from build123d import *

# Parameters (mm, degrees)
BOSS_EXTRUDE1_DEPTH       = 3.175
SKETCH2_R                 = 3.14
BOSS_EXTRUDE2_DEPTH       = 15.04125
F_4_CLEARANCE_HOLE1_D     = 3.2639
F_4_CLEARANCE_HOLE1_DEPTH = 25.4
F_4_CLEARANCE_HOLE1_TIP   = 0.980574487


with BuildPart() as part:
    # Sketch1 → Boss-Extrude1 (new body)
    with BuildSketch(Plane(origin=(0, 0, 0), x_dir=(1, 0, 0), z_dir=(0, 1, 0))):
        Polygon((0, 36.805), (-0.035, 36.805), (-52.035, 36.805), (-52.035, -36.805), (-0.035, -36.805), (0, -36.805), align=None)
    extrude(amount=-BOSS_EXTRUDE1_DEPTH)

    # Sketch2 → Boss-Extrude2 (add)
    with BuildSketch(Plane(origin=(0, 0, 0), x_dir=(1, 0, 0), z_dir=(0, 1, 0))):
        with BuildLine():
            Line((-3.175, 30.2), (0, 30.2))
            Line((0, 30.2), (0, 36.48))
            Line((0, 36.48), (-3.175, 36.48))
            ThreePointArc((-3.175, 36.48), (-6.315, 33.34), (-3.175, 30.2))
        make_face()
        with BuildLine():
            Line((-3.175, -36.48), (0, -36.48))
            Line((0, -36.48), (0, -30.2))
            Line((0, -30.2), (-3.175, -30.2))
            ThreePointArc((-3.175, -30.2), (-6.315, -33.34), (-3.175, -36.48))
        make_face()
        with Locations(Location((-48.895, 33.34, 0), (0, 0, 270))):
            Circle(SKETCH2_R)
        with Locations(Location((-48.895, -33.34, 0), (0, 0, 270))):
            Circle(SKETCH2_R)
    extrude(amount=-BOSS_EXTRUDE2_DEPTH)

    # #4 Clearance Hole1
    with Locations(Plane(origin=(0, -15.04125, 0), x_dir=(-1, 0, 0), z_dir=(0, -1, 0))):
        with Locations((48.895, 33.34), (3.175, 33.34), (3.175, -33.34), (48.895, -33.34)):
            Hole(F_4_CLEARANCE_HOLE1_D / 2, depth=F_4_CLEARANCE_HOLE1_DEPTH)
            with Locations((0, 0, -(F_4_CLEARANCE_HOLE1_DEPTH + F_4_CLEARANCE_HOLE1_TIP / 2))):  # 118° drill point
                Cone(0, F_4_CLEARANCE_HOLE1_D / 2, F_4_CLEARANCE_HOLE1_TIP, mode=Mode.SUBTRACT)

    # Mirror1: part across plane


with BuildPart() as part_1:
    add(part.part)
    add(part.part.mirror(Plane(origin=(0, -3.175, 0), x_dir=(0, 0, 1), z_dir=(-1, 0, 0))))


solid = part_1.part
The model under review builds one solid part; all positions refer to its coordinate system, in mm. A direction names the side the tool comes from. Round coordinates to 2 decimals unless told otherwise and drop trailing zeros. Write each loop counter-clockwise with the first axis right and the second up, starting at its lowest first coordinate (ties: lowest second). Pieces come first, ordered by that corner, then holes. Notation, with made-up numbers: M 83,7 L 136,7 A21 cw 136,39 Z; hole C 68,73 d1. An arc over 180 degrees is marked long. Use a Markdown table: item, result. Add a question column.
Q1. We need section C-C, the plane x = 11.5. State the section outline as (y, z) points (3 decimals).
Q2. The part is to be moulded in two halves that separate along X. For faces 6 (the face through (50.1, -7.42, 32.24)), 7 (the face through (52.035, -2, -1)), 8 (the face through (50.1, -9.03, 36.24)), 9 (the face through (0, -9, -36.48)), say which applies: pulls with the +X half, pulls with the -X half, needs draft (parallel to the pull), parting line crosses it, or undercut.
Q3. We need section B-B, the plane z = -7. State the section outline as (x, y) points (3 decimals), plus the area to 3 significant figures.
Q4. Machinability: for faces 1 (the face through (0, -9, -30.2)), 2 (the face through (-3.387, -7.415, 31.722)), 3 (the face through (0, -9, 36.48)), 4 (the face through (50, -15.041, 35)), 5 (the face through (6.314, -9.025, -33.409)), which of the approach directions +Z, -Z, +X, -X, +Y, -Y give a long, thin tool a straight path to every point of the face, cutting with its end or side? Answer none if there is none.
Q5. To check wall thickness, follow line 1 (X direction, y = -2.75, z = 33.34) (3 decimals); line 2 (Y direction, x = 27, z = 13) (3 decimals); line 3 (Z direction, x = 2, y = -12.25). State the ranges of each line that lie inside material, in increasing order.
Q6. Insertion check: pin 1 (2 mm diameter, centred on y = -8.5, z = -28.5, fed in from -X); pin 2 (5 mm diameter, centred on x = 0, y = -8, fed in from +Z); pin 3 (5 mm diameter, centred on x = -1, y = -6.5, fed in from -Z); pin 4 (4 mm diameter, centred on x = -28, z = 18.5, fed in from -Y) (3 decimals). Each pin has a flat end and moves straight along its axis. Give the tip position at first contact, or say it passes through.
Q7. We need section A-A, the plane y = -6.25. Count the separate pieces of the cut face and the enclosed holes in it, plus the area to 3 significant figures.
Findings below:
| question | item | result |
|---|---|---|
| 1 | outline | M -3.175,-36.805 L 0,-36.805 L 0,36.805 L -3.175,36.805 Z |
| 2 | face 6 | undercut |
| 2 | face 7 | pulls with the +X half |
| 2 | face 8 | undercut |
| 2 | face 9 | needs draft |
| 3 | outline | M -52.035,-3.175 L 52.035,-3.175 L 52.035,0 L -52.035,0 Z |
| 3 | area | 330 mm² |
| 4 | face 1 | +X, -X, -Y |
| 4 | face 2 | +Y, -Y |
| 4 | face 3 | +Z, +X, -X, -Y |
| 4 | face 4 | +Z, -Z, +X, -X, -Y |
| 4 | face 5 | -Y |
| 5 | line 1 | x = -52.035 to -50.527, -47.263 to -4.807, -1.543 to 1.543, 4.807 to 47.263, 50.527 to 52.035 |
| 5 | line 2 | y = -3.175 to 0 |
| 5 | line 3 | z = -36.48 to -34.47, -32.21 to -30.2, 30.2 to 32.21, 34.47 to 36.48 |
| 6 | pin 1 | passes through |
| 6 | pin 2 | stops at z = 36.48 |
| 6 | pin 3 | stops at z = -36.48 |
| 6 | pin 4 | stops at y = -3.175 |
| 7 | separate pieces | 6 |
| 7 | enclosed holes | 8 |
| 7 | area | 199 mm² |
